Read the model definition and answer for the solid it produces. Units are mm, in the model's axes. A direction names the side the tool comes from. Coordinates: 2 decimals unless noted, no trailing zeros. Write each loop counter-clockwise with the first axis right and the second up, starting at its lowest first coordinate (ties: lowest second). Pieces come first, ordered by that corner, then holes. Notation, with made-up numbers: M 20.25,40 L 29.25,40 A14 ccw 29.25,56 Z; hole C 56.25,10.25 d6. An arc over 180 degrees is marked long. Write item = value, one per line.
from build123d import *

# Parameters (mm, degrees)
SKETCH_11_W         = 15
SKETCH_11_H         = 15
SKETCH_11_W_2       = 13
SKETCH_11_H_2       = 13
F_15X15X1_1_DEPTH   = 100
SKETCH_12_R         = 1.6
CUT_EXTRUDE_1_DEPTH = 102.396498953


with BuildPart() as part:
    # 草图11 → 铝管 15X15X1(1) (new body)
    with BuildSketch(Plane(origin=(0, 0, 0), x_dir=(0, 0, -1), z_dir=(1, 0, 0))):
        Rectangle(SKETCH_11_W, SKETCH_11_H)
        Rectangle(SKETCH_11_W_2, SKETCH_11_H_2, mode=Mode.SUBTRACT)
    extrude(amount=F_15X15X1_1_DEPTH)

    # 草图12 → 切除-拉伸1 (cut, through all)
    with BuildSketch(Plane(origin=(0, 7.5, 0), x_dir=(1, 0, 0), z_dir=(0, 1, 0))):
        with Locations(Location((45, 0, 0), (0, 0, 270))):
            Circle(SKETCH_12_R)
        with Locations(Location((25, 0, 0), (0, 0, 270))):
            Circle(SKETCH_12_R)
        with Locations(Location((5, 0, 0), (0, 0, 270))):
            Circle(SKETCH_12_R)
    extrude(amount=-CUT_EXTRUDE_1_DEPTH, mode=Mode.SUBTRACT)


solid = part.part
Item 1: Find section A-A (z = 0). State how many separate pieces and enclosed holes the cut face has, and give its area (3 significant figures).
Worked answers:
separate_pieces = 8
enclosed_holes = 0
area = 181 mm²
Item 2: Which of the six approach directions +Z, -Z, +X, -X, +Y, -Y give full straight-line access (tool end or side, diameter ignored) to faces 4 (the face through (49, 0, -6.5)), 5 (the face through (43.58, 7.01, 0.74))?
Worked answers:
face_4 = +X, -X
face_5 = +Y, -Y
Item 3: Find section C-C (y = -3). Determine the outline of the cut face in (x, z).
Worked answers:
outline = M 0,-7.5 L 100,-7.5 L 100,-6.5 L 0,-6.5 Z; M 0,6.5 L 100,6.5 L 100,7.5 L 0,7.5 Z
Item 4: For a pull along Z with two mould halves and no side action, classify faces 1 (the face through (49, 0, 7.5)), 2 (the face through (49, -6.5, 0)), 3 (the face through (0, 0, 7)) as released by +Z, released by -Z, zero draft, split by the parting line, or undercut.
Worked answers:
face_1 = released by +Z
face_2 = undercut
face_3 = zero draft
Item 5: Find section D-D (x = 25). Determine the outline of the cut face in (y, z), and give its area (3 significant figures).
Worked answers:
outline = M -7.5,-7.5 L 7.5,-7.5 L 7.5,-1.6 L 6.5,-1.6 L 6.5,-6.5 L -6.5,-6.5 L -6.5,-1.6 L -7.5,-1.6 Z; M -7.5,1.6 L -6.5,1.6 L -6.5,6.5 L 6.5,6.5 L 6.5,1.6 L 7.5,1.6 L 7.5,7.5 L -7.5,7.5 Z
area = 49.6 mm²
Item 6: Find section B-B (x = 62.5). Determine the outline of the cut face in (y, z), and give its area (3 significant figures).
Worked answers:
outline = M -7.5,-7.5 L 7.5,-7.5 L 7.5,7.5 L -7.5,7.5 Z; hole M -6.5,-6.5 L 6.5,-6.5 L 6.5,6.5 L -6.5,6.5 Z
area = 56.0 mm²
Item 7: A flat-ended cylindrical pin translates along its axis: pin 1 (2.5 mm diameter, centred on x = 25, z = 0, fed in from +Y). Find the tip coordinate at first contact, or state that the pin passes through.
Worked answers:
pin_1 = through
Item 8: Consider line 1 along X through (y, z) = (6.7, 0); line 2 along Z through (x, y) = (39, -3.5). Determine where each line is inside the solid, lowest interval first. Write a range as from..to.
Worked answers:
line_1 = 0..3.4, 6.6..23.4, 26.6..43.4, 46.6..100
line_2 = -7.5..-6.5, 6.5..7.5
